Here's how the part is built. I have some questions about the finished solid (model axes, mm). A direction names the side the tool comes from. Give positions to 0.01 mm unless a question says otherwise; leave off trailing zeros. Write each loop counter-clockwise with the first axis right and the second up, starting at its lowest first coordinate (ties: lowest second). Pieces come first, ordered by that corner, then holes. Notation, with made-up numbers: (39, 31.5) - (94, 31.5) arc R11 ccw to (94, 42.5) - close; hole circle Ø6 at (23.5, 50). An arc over 180 degrees is marked (long way). Use a Markdown table: item, result.
```python
from build123d import *

# Parameters (mm, degrees)
BOSS_EXTRUDE1_DEPTH     = 25.4
CUT_EXTRUDE1_START      = -6.35
CUT_EXTRUDE1_DEPTH      = 107.95
SKETCH3_W               = 44.45
SKETCH3_H               = 25.4
BOSS_EXTRUDE2_DEPTH     = 6.35
BOSS_EXTRUDE3_START     = -120.65
SKETCH3_2_W             = 44.45
SKETCH3_2_H             = 25.4
BOSS_EXTRUDE3_DEPTH     = 6.35
BOSS_EXTRUDE4_START     = -25.4
SKETCH8_W               = 6.35
SKETCH8_H               = 12.7
BOSS_EXTRUDE4_DEPTH     = 38.1
CUT_EXTRUDE2_DEPTH      = 206.865393886
CUT_EXTRUDE2_DEPTH_BACK = 206.865393886
SKETCH9_R               = 3.2385
SKETCH10_R              = 1.000000032
CUT_EXTRUDE3_DEPTH      = 183.990209847


with BuildPart() as part:
    # Sketch1 → Boss-Extrude1 (new body)
    with BuildSketch(Plane(origin=(0, 0, 0), x_dir=(1, 0, 0), z_dir=(0, 1, 0))):
        Polygon((3.175, 114.3), (0, 114.3), (0, 120.65), (119.38, 120.65), (119.38, 0), (0, 0), (0, 6.35), (3.175, 6.35), (113.03, 6.35), (113.03, 114.3), align=None)
    extrude(amount=BOSS_EXTRUDE1_DEPTH)

    # Sketch2 → Cut-Extrude1 (cut)
    with BuildSketch(Plane.XY.offset(CUT_EXTRUDE1_START)):
        Polygon((119.38, 25.4), (113.03, 24.13), (113.03, 25.4), align=None)
    extrude(amount=-CUT_EXTRUDE1_DEPTH, mode=Mode.SUBTRACT)

    # Sketch3 → Boss-Extrude2 (add)
    with BuildSketch(Plane.XY):
        with Locations((-15.875, 12.7)):
            Rectangle(SKETCH3_W, SKETCH3_H)
    extrude(amount=BOSS_EXTRUDE2_DEPTH)

    # Sketch3<2> → Boss-Extrude3 (add)
    with BuildSketch(Plane.XY.offset(BOSS_EXTRUDE3_START)):
        with Locations((-15.875, 12.7)):
            Rectangle(SKETCH3_2_W, SKETCH3_2_H)
    extrude(amount=-BOSS_EXTRUDE3_DEPTH)

    # Sketch8 → Boss-Extrude4 (add)
    with BuildSketch(Plane(origin=(0, 25.4, 0), x_dir=(1, 0, 0), z_dir=(0, 1, 0)).offset(BOSS_EXTRUDE4_START)):
        with Locations((116.205, 0)):
            Rectangle(SKETCH8_W, SKETCH8_H)
        with Locations((3.175, 0)):
            Rectangle(SKETCH8_W, SKETCH8_H)
        with Locations((3.175, 120.65)):
            Rectangle(SKETCH8_W, SKETCH8_H)
        with Locations((116.205, 120.65)):
            Rectangle(SKETCH8_W, SKETCH8_H)
    extrude(amount=BOSS_EXTRUDE4_DEPTH)

    # Sketch9 → Cut-Extrude2 (cut, two sides: drawn at the far end of the back side and taken through both)
    with BuildSketch(Plane(origin=(119.38, 0, 0), x_dir=(0, 0, -1), z_dir=(1, 0, 0)).offset(-CUT_EXTRUDE2_DEPTH_BACK)):
        with Locations((0, 31.75)):
            Circle(SKETCH9_R)
        with Locations((120.65, 31.75)):
            Circle(SKETCH9_R)
    extrude(amount=CUT_EXTRUDE2_DEPTH + CUT_EXTRUDE2_DEPTH_BACK, mode=Mode.SUBTRACT)

    # Sketch10 → Cut-Extrude3 (cut, through all)
    with BuildSketch(Plane.XY.offset(6.35)):
        with Locations((-25.4, 22.225)):
            Circle(SKETCH10_R)
        with Locations((-25.4, 3.175)):
            Circle(SKETCH10_R)
    extrude(amount=-CUT_EXTRUDE3_DEPTH, mode=Mode.SUBTRACT)


solid = part.part
```
Item 1: Will these pins go through, and if not, where does the flat tip stop? pin 1 Ø1.9 at (x, z) = (77.5, -1.5) entering from +Y; pin 2 Ø1.6 at (x, y) = (-25.4, 22.225) entering from +Z; pin 3 Ø12.5 at (x, y) = (63.5, 17) entering from +Z; pin 4 Ø3 at (y, z) = (11.5, -18) entering from -X.
Values:
| item | result |
|---|---|
| pin 1 | stops at y = 25.4 |
| pin 2 | passes through |
| pin 3 | stops at z = 0 |
| pin 4 | stops at x = 113.03 |
Item 2: I need wall thicknesses on line 1 along Z through (x, y) = (2.75, 31.75); line 2 along Y through (x, z) = (-25.4, -123.5) (3 decimals); line 3 along Y through (x, z) = (115, -120.65). Which ranges of each line are inside material? Lowest first, please. Write a range as [from, to].
Values:
| item | result |
|---|---|
| line 1 | z = [-127, -123.89], [-117.41, -114.3], [-6.35, -3.24], [3.24, 6.35] |
| line 2 | y = [0, 2.175], [4.175, 21.225], [23.225, 25.4] |
| line 3 | y = [0, 28.51], [34.99, 38.1] |
Item 3: Thinking about a two-plate mould opening in X: for faces 4 (the flat face through (116.249, 24.774, -59.569)), 5 (the flat face through (59, 25.4, -117)), 6 (the cylindrical face through (3.13, 30.51, -123.64)), which applies, +X half, -X half, draft (parallel to the pull), parting line (faces both ways), or undercut?
Values:
| item | result |
|---|---|
| face 4 | -X half |
| face 5 | undercut |
| face 6 | draft |
Item 4: For faces 1 (the flat face through (-19, 13, 0)), 2 (the flat face through (60, 13, 0)), 3 (the flat face through (59, 25.4, -3)), which set-ups out of +Z, -Z, +X, -X, +Y, -Y let a thin tool reach every point of the face, with its end or its side?
Values:
| item | result |
|---|---|
| face 1 | -X, +Y, -Y |
| face 2 | +Z, +Y, -Y |
| face 3 | +Z, -Z, +Y |
Item 5: If we section it at D-D, the plane z = -36.5: Write out the boundary of the cut face in (x, y), plus the area to 3 significant figures.
Values:
| item | result |
|---|---|
| outline | (113.03, 0) - (119.38, 0) - (119.38, 25.4) - (113.03, 24.13) - close |
| area | 157 mm2 |
Item 6: If we section it at B-B, the plane y = 31.75: Count the separate pieces of the cut face and the enclosed holes in it, plus the area to 3 significant figures.
Values:
| item | result |
|---|---|
| separate pieces | 8 |
| enclosed holes | 0 |
| area | 158 mm2 |
Item 7: If we section it at C-C, the plane y = 10: Write out the boundary of the cut face in (x, z).
Values:
| item | result |
|---|---|
| outline | (-38.1, -127) - (6.35, -127) - (6.35, -120.65) - (113.03, -120.65) - (113.03, -127) - (119.38, -127) - (119.38, 6.35) - (113.03, 6.35) - (113.03, 0) - (6.35, 0) - (6.35, 6.35) - (-38.1, 6.35) - (-38.1, 0) - (0, 0) - (0, -6.35) - (113.03, -6.35) - (113.03, -114.3) - (0, -114.3) - (0, -120.65) - (-38.1, -120.65) - close |
Item 8: If we section it at A-A, the plane x = 71.5: Write out the boundary of the cut face in (y, z).
Values:
| item | result |
|---|---|
| outline | (0, -120.65) - (25.4, -120.65) - (25.4, -114.3) - (0, -114.3) - close; (0, -6.35) - (25.4, -6.35) - (25.4, 0) - (0, 0) - close |
